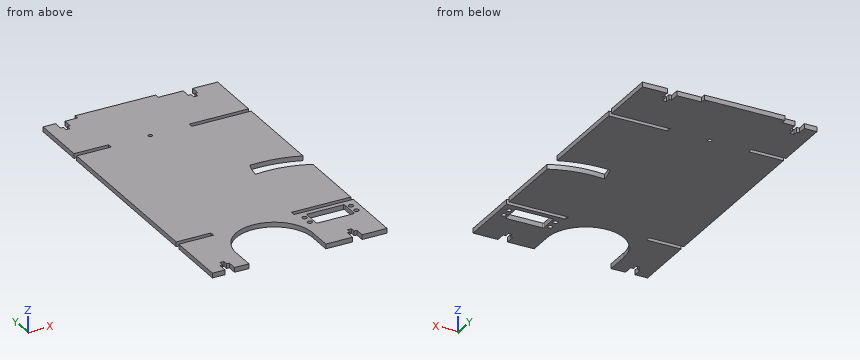
from build123d import *

# Parameters (mm, degrees)
SKETCH2_W           = 184
SKETCH2_H           = 332.5
BOSS_EXTRUDE1_DEPTH = 5
SKETCH3_W           = 36.5
SKETCH3_H           = 5
SKETCH3_W_2         = 62.5
CUT_EXTRUDE1_DEPTH  = 5
CUT_EXTRUDE2_DEPTH  = 10
SKETCH5_R           = 2.1
CUT_EXTRUDE3_DEPTH  = 10
SKETCH6_R           = 2.5
CUT_EXTRUDE4_DEPTH  = 20
CUT_EXTRUDE6_DEPTH  = 6


with BuildPart() as part:
    # Sketch2 → Boss-Extrude1 (new body)
    with BuildSketch(Plane.XY):
        Rectangle(SKETCH2_W, SKETCH2_H)
    extrude(amount=BOSS_EXTRUDE1_DEPTH)

    # Sketch3 → Cut-Extrude1 (cut)
    with BuildSketch(Plane.XY.offset(5)):
        with Locations((-73.75, -98.75)):
            Rectangle(SKETCH3_W, SKETCH3_H)
        with Locations((60.75, -98.75)):
            Rectangle(SKETCH3_W_2, SKETCH3_H)
        with Locations((-73.75, 163.75)):
            Rectangle(SKETCH3_W, SKETCH3_H)
        with Locations((60.75, 163.75)):
            Rectangle(SKETCH3_W_2, SKETCH3_H)
        with Locations((60.75, 98.75)):
            Rectangle(SKETCH3_W_2, SKETCH3_H)
        with BuildLine():
            Line((27.5, -141.25), (27.5, -166.25))
            Line((27.5, -166.25), (-53.5, -166.25))
            Line((-53.5, -166.25), (-53.5, -141.25))
            ThreePointArc((-53.5, -141.25), (-13, -100.75), (27.5, -141.25))
        make_face()
        with Locations((-73.75, 98.75)):
            Rectangle(SKETCH3_W, SKETCH3_H)
    extrude(amount=-CUT_EXTRUDE1_DEPTH, mode=Mode.SUBTRACT)

    # Sketch4 → Cut-Extrude2 (cut)
    with BuildSketch(Plane.XY.offset(5)):
        Polygon((55.75, 161.25), (55.75, 151.25), (58.65, 151.25), (58.65, 146.25), (62.85, 146.25), (62.85, 151.25), (65.75, 151.25), (65.75, 161.25), align=None)
        Polygon((-78.75, 161.25), (-78.75, 151.25), (-75.85, 151.25), (-75.85, 146.25), (-71.65, 146.25), (-71.65, 151.25), (-68.75, 151.25), (-68.75, 161.25), align=None)
        Polygon((65.75, -166.25), (65.75, -156.25), (62.85, -156.25), (62.85, -151.25), (58.65, -151.25), (58.65, -156.25), (55.75, -156.25), (55.75, -166.25), align=None)
        Polygon((-68.75, -166.25), (-68.75, -156.25), (-71.65, -156.25), (-71.65, -151.25), (-75.85, -151.25), (-75.85, -156.25), (-78.75, -156.25), (-78.75, -166.25), align=None)
    extrude(amount=-CUT_EXTRUDE2_DEPTH, mode=Mode.SUBTRACT)

    # Sketch5 → Cut-Extrude3 (cut)
    with BuildSketch(Plane.XY.offset(5)):
        with Locations((-13, 98.75)):
            Circle(SKETCH5_R)
    extrude(amount=-CUT_EXTRUDE3_DEPTH, mode=Mode.SUBTRACT)

    # Sketch6 → Cut-Extrude4 (cut)
    with BuildSketch(Plane(origin=(0, 0, 0), x_dir=(-1, 0, 0), z_dir=(0, 0, -1))):
        with Locations((-35.2, -111.17)):
            Circle(SKETCH6_R)
        with Locations((-35.2, -121.33)):
            Circle(SKETCH6_R)
        with Locations((-84.2, -111.17)):
            Circle(SKETCH6_R)
        with Locations((-84.2, -121.33)):
            Circle(SKETCH6_R)
        with BuildLine():
            Line((-78.2, -106.25), (-41.2, -106.25))
            Line((-41.2, -106.25), (-40.7, -106.25))
            ThreePointArc((-40.7, -106.25), (-39.992893219, -106.542893219), (-39.7, -107.25))
            Line((-39.7, -107.25), (-39.7, -125.25))
            ThreePointArc((-39.7, -125.25), (-39.992893219, -125.957106781), (-40.7, -126.25))
            Line((-40.7, -126.25), (-78.7, -126.25))
            ThreePointArc((-78.7, -126.25), (-79.407106781, -125.957106781), (-79.7, -125.25))
            Line((-79.7, -125.25), (-79.7, -107.25))
            ThreePointArc((-79.7, -107.25), (-79.407106781, -106.542893219), (-78.7, -106.25))
            Line((-78.7, -106.25), (-78.2, -106.25))
        make_face()
    extrude(amount=-CUT_EXTRUDE4_DEPTH, mode=Mode.SUBTRACT)

    # Sketch7 → Cut-Extrude6 (cut, through all)
    with BuildSketch(Plane.XY.offset(5)):
        with BuildLine():
            Line((92.018319465, -3.95948465), (92, -22.885338591))
            ThreePointArc((92, -22.885338591), (64.618518363, -14.841480585), (36.080546525, -14.658856257))
            ThreePointArc((36.080546525, -14.658856257), (37.397553955, -5.515336457), (39.976105832, 3.355375641))
            ThreePointArc((39.976105832, 3.355375641), (66.402572717, 2.581915177), (92.018319465, -3.95948465))
        make_face()
    extrude(amount=-CUT_EXTRUDE6_DEPTH, mode=Mode.SUBTRACT)


solid = part.part
Read the model definition and answer for the solid it produces. Units are mm, in the model's axes. Round coordinates to 2 decimals unless told otherwise and drop trailing zeros. Loops run counter-clockwise (first coordinate to the right, second up) from the corner with the lowest first, then second, coordinate; pieces in that order, holes last.
Q1. Section C-C on x = -37.5 is taken. Write down the section's boundary in (y, z), and give its area (3 significant figures).
Q2. Each of these flat-tipped pins is pushed along its axis until it touches: pin 1 (2.5 mm diameter, centred on x = -62.5, z = 3, fed in from +Y); pin 2 (2 mm diameter, centred on x = 60, z = 3, fed in from -Y); pin 3 (3 mm diameter, centred on x = -70.5, z = 1.5, fed in from +Y). Where does it stop, or does it pass through?
Q3. Section B-B on z = 2.6 is taken. Give the number of separate pieces and of enclosed holes in the cut face, and give its area (3 significant figures).
Q4. Consider probe 1 along X at (y, z) = (-152, 1.1); probe 2 along Y at (x, z) = (46, 2.9); probe 3 along Y at (x, z) = (-72, 1.5). Determine where each line is inside the solid, lowest interval first.
Q5. Section A-A on x = -63.5 is taken. Write down the section's boundary in (y, z), and give its area (3 significant figures).
Output:
1. outline: (-109, 0) - (166.25, 0) - (166.25, 5) - (-109, 5) - close
1. area: 1,380 mm2
2. pin 1: stops at y = 161.25
2. pin 2: stops at y = -151.25
2. pin 3: stops at y = 151.25
3. separate pieces: 1
3. enclosed holes: 6
3. area: 52,700 mm2
4. probe 1: x = -92 to -75.85, -71.65 to -53.5, 27.5 to 58.65, 62.85 to 92
4. probe 2: y = -166.25 to -126.25, -106.25 to -101.25, -96.25 to -13.82, 3.69 to 96.25, 101.25 to 161.25
4. probe 3: y = -151.25 to -101.25, -96.25 to 96.25, 101.25 to 146.25
5. outline: (-166.25, 0) - (-101.25, 0) - (-101.25, 5) - (-166.25, 5) - close; (-96.25, 0) - (96.25, 0) - (96.25, 5) - (-96.25, 5) - close; (101.25, 0) - (161.25, 0) - (161.25, 5) - (101.25, 5) - close
5. area: 1,590 mm2
